from build123d import *

# Parameters (mm, degrees)
ESQUISSE1_R                  = 5
BOSS_EXTRU_1_DEPTH           = 600
ESQUISSE2_R                  = 10
BOSS_EXTRU_2_DEPTH           = 200
CHANFREIN1_SIZE              = 10
CHANFREIN1_SIZE_2            = 286.362532829
ESQUISSE3_R                  = 4
ENL_V_MAT_EXTRU_1_DEPTH      = 601.166643525
ESQUISSE4_R                  = 8
ESQUISSE4_R_2                = 4.5
BOSS_EXTRU_3_DEPTH           = 3
ESQUISSE5_R                  = 6
BOSS_EXTRU_4_DEPTH           = 25
ENL_V_MAT_EXTRU_2_DEPTH      = 601.733718055
ENL_V_MAT_EXTRU_2_DEPTH_BACK = 601.733718055
ESQUISSE6_W                  = 10
ESQUISSE6_H                  = 13.340291415
ESQUISSE7_R                  = 1.5
ENL_V_MAT_EXTRU_3_DEPTH      = 603.292287858


with BuildPart() as part:
    # Esquisse1 → Boss.-Extru.1 (new body)
    with BuildSketch(Plane(origin=(0, 0, 0), x_dir=(1, 0, 0), z_dir=(0, 1, 0))):
        with Locations(Location((0, 0, 0), (0, 0, 270))):
            Circle(ESQUISSE1_R)
    extrude(amount=BOSS_EXTRU_1_DEPTH)

    # Esquisse2 → Boss.-Extru.2 (add)
    with BuildSketch(Plane(origin=(0, 0, 0), x_dir=(1, 0, 0), z_dir=(0, 1, 0))):
        with Locations(Location((0, 0, 0), (0, 0, 90))):
            Circle(ESQUISSE2_R)
    extrude(amount=BOSS_EXTRU_2_DEPTH)

    # Chanfrein1
    # the kernel refuses this chamfer: 286.362532829, 10 mm, written as the material it adds along each edge
    with BuildSketch(Plane(origin=(0, 200, 0), x_dir=(0, 0, 1), z_dir=(1, 0, 0))) as chanfrein1_piece_1_section:
        Polygon((5 + CHANFREIN1_SIZE, 0), (5, -CHANFREIN1_SIZE_2), (5, 0), align=None)
    chanfrein1_piece_1 = revolve(axis=Axis((0, 200, 0), (0, -1, 0)), mode=Mode.PRIVATE)
    chanfrein1_piece_1 = chanfrein1_piece_1 & Plane(origin=(0, 318.034394442, 0), x_dir=(0, 0, -1), z_dir=(0, -1, 0)) * Cylinder(10, 1146, mode=Mode.PRIVATE)
    add(chanfrein1_piece_1)

    # Esquisse3 → Enlèv. mat.-Extru.1 (cut, through all)
    with BuildSketch(Plane(origin=(0, 600, 0), x_dir=(1, 0, 0), z_dir=(0, 1, 0))):
        with Locations(Location((0, 0, 0), (0, 0, 270))):
            Circle(ESQUISSE3_R)
    extrude(amount=-ENL_V_MAT_EXTRU_1_DEPTH, mode=Mode.SUBTRACT)

    # Esquisse4 → Boss.-Extru.3 (add)
    with BuildSketch(Plane(origin=(0, 590, 0), x_dir=(1, 0, 0), z_dir=(0, 1, 0))):
        with Locations(Location((0, 0, 0), (0, 0, 270))):
            Circle(ESQUISSE4_R)
        Circle(ESQUISSE4_R_2, mode=Mode.SUBTRACT)
    extrude(amount=BOSS_EXTRU_3_DEPTH)

    # Esquisse5 → Boss.-Extru.4 (add, symmetric)
    with BuildSketch(Plane.XY):
        with Locations((-10, 0)):
            Circle(ESQUISSE5_R)
    extrude(amount=BOSS_EXTRU_4_DEPTH, both=True)

    # Esquisse6 → Enlèv. mat.-Extru.2 (cut, two sides: drawn at the far end of the back side and taken through both)
    with BuildSketch(Plane(origin=(0, 0, 0), x_dir=(0, 0, -1), z_dir=(1, 0, 0)).offset(-ENL_V_MAT_EXTRU_2_DEPTH_BACK)):
        with Locations((-10, -6.670145708)):
            Rectangle(ESQUISSE6_W, ESQUISSE6_H)
        with Locations((10, -6.670145708)):
            Rectangle(ESQUISSE6_W, ESQUISSE6_H)
    extrude(amount=ENL_V_MAT_EXTRU_2_DEPTH + ENL_V_MAT_EXTRU_2_DEPTH_BACK, mode=Mode.SUBTRACT)

    # Esquisse7 → Enlèv. mat.-Extru.3 (cut, through all)
    with BuildSketch(Plane.XY.offset(25)):
        with Locations((-10, 0)):
            Circle(ESQUISSE7_R)
    extrude(amount=-ENL_V_MAT_EXTRU_3_DEPTH, mode=Mode.SUBTRACT)


solid = part.part
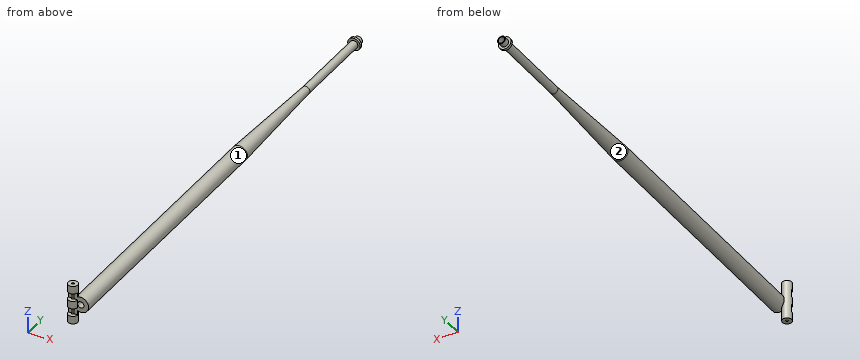
The listing builds one solid part. Answer for the finished solid, in the listing's coordinates (mm). Face numbers are marked on the shaded views. Round coordinates to 2 decimals unless told otherwise and drop trailing zeros. Write each loop counter-clockwise with the first axis right and the second up, starting at its lowest first coordinate (ties: lowest second). Pieces come first, ordered by that corner, then holes. Notation, with made-up numbers: (16.25, 3) - (65.25, 3) arc R7 cw to (65.25, 7) - close; hole circle Ø5 at (31.25, 28). An arc over 180 degrees is marked (long way). Use one line per item in the form item = value. Start each with the question number.
Item 1: A cutting plane is placed at B-B (y = 563.5). Write down the section's boundary in (x, z).
Item 2: Find the intervals of material crossed by line 1 (Z direction, x = 0, y = 319); line 2 (Y direction, x = -10, z = 13); line 3 (X direction, y = 76.5, z = 8), in increasing order. Write a range as [from, to].
Item 3: Flat-ended cylindrical pins translate along their axes: pin 1 Ø3.5 at (x, z) = (-13, 10) entering from -Y; pin 2 Ø8 at (x, z) = (4.5, -8.5) entering from +Y; pin 3 Ø10 at (y, z) = (439, 7.5) entering from -X. Find the tip coordinate at first contact, or state that the pin passes through.
Item 4: A cutting plane is placed at A-A (x = 0). Write down the section's boundary in (y, z), plus the area to 3 significant figures.
Item 5: A cutting plane is placed at C-C (y = 373.5). Write down the section's boundary in (x, z), plus the area to 3 significant figures.
Item 6: Determine the mould class of the marked faces 1 and 2 for opening direction Y: +Y half, -Y half, draft (parallel to the pull), parting line (faces both ways), or undercut.
The answers:
q1.outline = circle Ø10 at (0, 0); hole circle Ø8 at (0, 0)
q2.line_1 = [-10, -4], [4, 10]
q2.line_2 = [1.5, 6]
q2.line_3 = [-6, 6]
q3.pin_1 = 0
q3.pin_2 = 593
q3.pin_3 = -6.18
q4.outline = (0, -10) - (343.18, -10) - (486.36, -5) - (590, -5) - (590, -8) - (593, -8) - (593, -5) - (600, -5) - (600, -4) - (0, -4) - close; (0, 4) - (600, 4) - (600, 5) - (593, 5) - (593, 8) - (590, 8) - (590, 5) - (486.36, 5) - (343.18, 10) - (0, 10) - close
q4.area = 5,370 mm^2
q5.outline = circle Ø17.88 at (0, 0); hole circle Ø8 at (0, 0)
q5.area = 201 mm^2
q6.face_1 = draft
q6.face_2 = undercut
